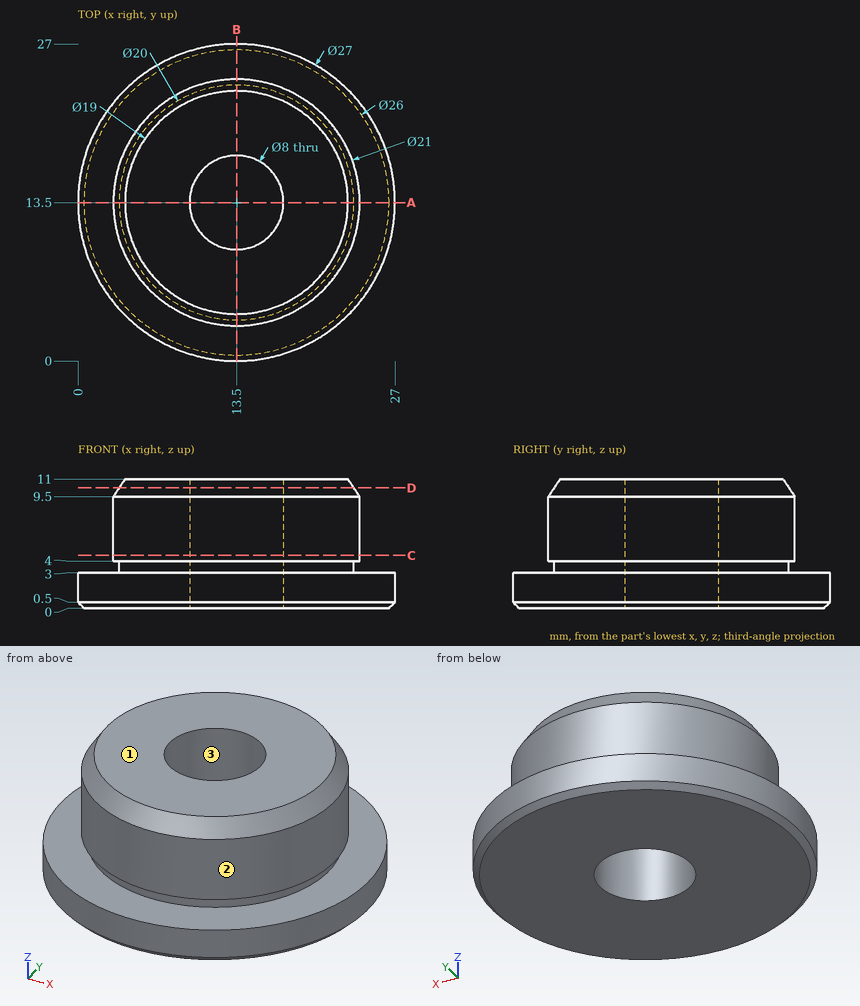
Part print with two shaded views. Sizes in mm from the minimum x, y, z corner. Give positions to 0.01 mm unless a question says otherwise; leave off trailing zeros. Order: outer loops, then holes, each group sorted by start corner. A loop starts at its lowest first (then second) coordinate and runs counter-clockwise, first axis right, second up.
(1) Drill centre lines: L1, parallel to Y at x = 13.5, z = 3.5; L2, parallel to Y at x = 13.5, z = 7.25; L3, parallel to Z at x = 18.25, y = 24. Where is each one in solid material? Low to high.
(2) Mould opens along X. For the marked faces 1, 2 and 3 say: released by +X, released by -X, zero draft, split by the parting line, or undercut.
(3) Saw through at A-A, the plane y = 13.5. Give the cut face in (x, z).
(4) Flat gauge pins, fed straight in: pin 1 (5 mm diameter, centred on x = 8, z = 2.5, fed in from +Y); pin 2 (6 mm diameter, centred on x = 10.5, z = 8, fed in from +Y); pin 3 (10.5 mm diameter, centred on x = 13.5, y = 13.5, fed in from -Z). Where does each tip first touch, or does it go through?
(5) Saw through at D-D, the plane z = 10.25. Give the cut face in (x, y).
(6) Saw through at C-C, the plane z = 4.5. Give the cut face in (x, y), then the cut area to 3 significant figures.
Results found:
1. L1: y = 3.5 to 9.5, 17.5 to 23.5
1. L2: y = 3 to 9.5, 17.5 to 24
1. L3: z = 0 to 3
2. face 1: zero draft
2. face 2: split by the parting line
2. face 3: undercut
3. outline: (0, 0.5) - (0.5, 0) - (9.5, 0) - (9.5, 11) - (4, 11) - (3, 9.5) - (3, 4) - (3.5, 4) - (3.5, 3) - (0, 3) - close; (17.5, 0) - (26.5, 0) - (27, 0.5) - (27, 3) - (23.5, 3) - (23.5, 4) - (24, 4) - (24, 9.5) - (23, 11) - (17.5, 11) - close
4. pin 1: stops at y = 26.66
4. pin 2: stops at y = 24
4. pin 3: stops at z = 0
5. outline: circle Ø20 at (13.5, 13.5); hole circle Ø8 at (13.5, 13.5)
6. outline: circle Ø21 at (13.5, 13.5); hole circle Ø8 at (13.5, 13.5)
6. area: 296 mm2
